```python
from build123d import *

# Parameters (mm, degrees)
CROQUIS1_W              = 82
CROQUIS1_H              = 90.5
CROQUIS1_R              = 1.4
SALIENTE_EXTRUIR1_DEPTH = 1.5
CROQUIS1_3_W            = 82
CROQUIS1_3_H            = 2
SALIENTE_EXTRUIR2_DEPTH = 9.31
SALIENTE_EXTRUIR3_START = 9.31
CROQUIS1_4_W            = 82
CROQUIS1_4_H            = 7.5
CROQUIS1_4_R            = 1.4
CROQUIS1_4_H_2          = 2
SALIENTE_EXTRUIR3_DEPTH = 2
CROQUIS2_R              = 1.5
CROQUIS2_R_2            = 1.6
CORTAR_EXTRUIR1_DEPTH   = 1.5
CROQUIS3_W              = 48
CROQUIS3_H              = 7.5
CORTAR_EXTRUIR2_DEPTH   = 87.58467604
REDONDEO1_R             = 5
REDONDEO2_R             = 3


with BuildPart() as part:
    # Croquis1 → Saliente-Extruir1 (new body)
    with BuildSketch(Plane(origin=(0, 0, 0), x_dir=(1, 0, 0), z_dir=(0, 1, 0))):
        with Locations((2.5, 28.755)):
            Rectangle(CROQUIS1_W, CROQUIS1_H)
        with Locations(Location((-25.63, 31.995, 0), (0, 0, 270))):
            Circle(CROQUIS1_R, mode=Mode.SUBTRACT)
        with Locations(Location((25.63, 31.995, 0), (0, 0, 270))):
            Circle(CROQUIS1_R, mode=Mode.SUBTRACT)
    extrude(amount=SALIENTE_EXTRUIR1_DEPTH)

    # Croquis2 → Cortar-Extruir1 (cut)
    with BuildSketch(Plane(origin=(0, 1.5, 0), x_dir=(1, 0, 0), z_dir=(0, 1, 0))):
        with Locations(Location((-23.4, -1.495, 0), (0, 0, 270))):
            Circle(CROQUIS2_R)
        with Locations(Location((23.4, -1.495, 0), (0, 0, 270))):
            Circle(CROQUIS2_R)
        with Locations(Location((0, 30.505, 0), (0, 0, 270))):
            Circle(CROQUIS2_R)
        with Locations(Location((-20.86, 57.715, 0), (0, 0, 270))):
            Circle(CROQUIS2_R_2)
        with Locations(Location((20.86, 57.715, 0), (0, 0, 270))):
            Circle(CROQUIS2_R_2)
        with Locations(Location((20.86, 15.995, 0), (0, 0, 270))):
            Circle(CROQUIS2_R_2)
        with Locations(Location((-20.86, 15.995, 0), (0, 0, 270))):
            Circle(CROQUIS2_R_2)
    extrude(amount=-CORTAR_EXTRUIR1_DEPTH, mode=Mode.SUBTRACT)


with BuildPart() as body_2:
    # Croquis1<3> → Saliente-Extruir2 (new body)
    with BuildSketch(Plane(origin=(0, 0, 0), x_dir=(1, 0, 0), z_dir=(0, 1, 0))):
        with Locations((2.5, -17.495)):
            Rectangle(CROQUIS1_3_W, CROQUIS1_3_H)
    extrude(amount=SALIENTE_EXTRUIR2_DEPTH)

    # Croquis1<4> → Saliente-Extruir3 (add)
    # profile 1 of 2: a face of its own
    with BuildSketch(Plane(origin=(0, 0, 0), x_dir=(1, 0, 0), z_dir=(0, 1, 0)).offset(SALIENTE_EXTRUIR3_START)):
        with Locations((2.5, -22.245)):
            Rectangle(CROQUIS1_4_W, CROQUIS1_4_H)
        with Locations(Location((-19, -21.995, 0), (0, 0, 270))):
            Circle(CROQUIS1_4_R, mode=Mode.SUBTRACT)
        with Locations(Location((39, -21.995, 0), (0, 0, 270))):
            Circle(CROQUIS1_4_R, mode=Mode.SUBTRACT)
    # profile 2 of 2: a face of its own
    with BuildSketch(Plane(origin=(0, 0, 0), x_dir=(1, 0, 0), z_dir=(0, 1, 0)).offset(SALIENTE_EXTRUIR3_START)):
        with Locations((2.5, -17.495)):
            Rectangle(CROQUIS1_4_W, CROQUIS1_4_H_2)
    extrude(amount=SALIENTE_EXTRUIR3_DEPTH)

    # Combinar1: union part
    add(part.part)

    # Croquis3 → Cortar-Extruir2 (cut, through all)
    with BuildSketch(Plane(origin=(0, 11.31, 0), x_dir=(1, 0, 0), z_dir=(0, 1, 0))):
        Polygon((-18.5, -25.995), (-28, -16.495), (-38.5, -16.495), (-38.5, -25.995), align=None)
        Polygon((-28, -16.495), (-38.5, -5.995), (-38.5, -16.495), align=None)
        with Locations((10.5, -22.245)):
            Rectangle(CROQUIS3_W, CROQUIS3_H)
        Polygon((-38.5, 54.005), (-18.5, 74.005), (-38.5, 74.005), align=None)
        Polygon((23.5, 74.005), (43.5, 54.005), (43.5, 74.005), align=None)
    extrude(amount=-CORTAR_EXTRUIR2_DEPTH, mode=Mode.SUBTRACT)

    # Redondeo1
    redondeo1_edges = [body_2.edges().sort_by_distance(p)[0] for p in [
        (23.5, 0.75, -74.005),
        (43.5, 0.75, -54.005),
        (-38.5, 0.75, 5.995),
        (-18.5, 0.75, -74.005),
        (-38.5, 0.75, -54.005),
    ]]
    fillet(redondeo1_edges, radius=REDONDEO1_R)

    # Redondeo2
    redondeo2_edges = [body_2.edges().sort_by_distance(p)[0] for p in [
        (-18.5, 10.31, 25.995),
        (43.5, 10.31, 25.995),
        (34.5, 10.31, 18.495),
        (-13.5, 10.31, 25.995),
        (-13.5, 10.31, 18.495),
        (34.5, 10.31, 25.995),
    ]]
    fillet(redondeo2_edges, radius=REDONDEO2_R)


solid = body_2.part
```
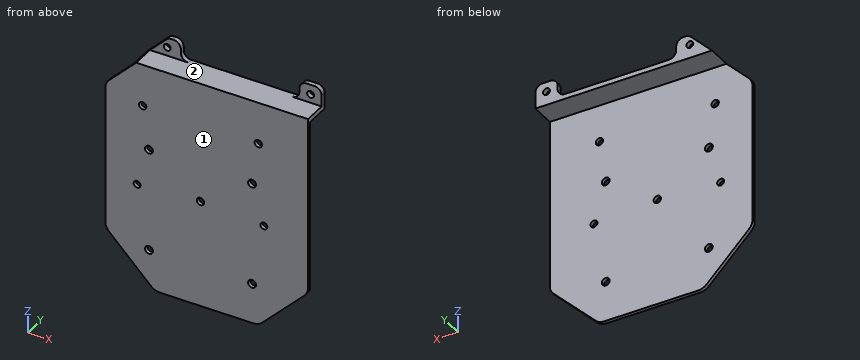
Input: part model. Units: mm. Frame: model coordinates. Face numbers are marked on the shaded views. Give positions to 0.01 mm unless a question says otherwise; leave off trailing zeros. Order: outer loops, then holes, each group sorted by start corner. A loop starts at its lowest first (then second) coordinate and runs counter-clockwise, first axis right, second up.
1. Cut plane A-A (x = 39). Return loops of the section in (y, z) (3 decimals).
Computed:
outline: (0, -58.505) - (1.5, -58.505) - (1.5, 16.495) - (11.31, 16.495) - (11.31, 20.595) - (9.31, 20.595) - (9.31, 18.495) - (0, 18.495) - close; (9.31, 23.395) - (11.31, 23.395) - (11.31, 25.995) - (9.31, 25.995) - close
2. Pin query (flat end, axial travel): pin 1 Ø3 at (x, z) = (-20.86, -15.995) entering from -Y; pin 2 Ø4.5 at (x, z) = (39, 21.995) entering from -Y; pin 3 Ø3 at (x, y) = (3, 9.5) entering from +Z (3 decimals); pin 4 Ø0.8 at (y, z) = (10.5, 22.5) entering from -X (3 decimals). Return the tip coordinate at first contact, or that it passes through.
Computed:
pin 1: passes through
pin 2: stops at y = 9.31
pin 3: stops at z = 18.495
pin 4: stops at x = -22.395
3. Cut plane D-D (y = 6.75). Return loops of the section in (x, z) (3 decimals), and give its area (3 significant figures).
Computed:
outline: (-28, 16.495) - (43.5, 16.495) - (43.5, 18.495) - (-26, 18.495) - close
area: 141 mm2
4. Cut plane C-C (z = -38). Return loops of the section in (x, y).
Computed:
outline: (-38.5, 0) - (43.5, 0) - (43.5, 1.5) - (-38.5, 1.5) - close
5. Draft query along X for the marked faces 1 and 2. Return one class per face: released by +X, released by -X, zero draft, split by the parting line, or undercut.
Computed:
face 1: zero draft
face 2: undercut
6. Line query: probe 1 along Z at (x, y) = (-25, 8) (3 decimals); probe 2 along Y at (x, z) = (-20.5, -55.5); probe 3 along X at (y, z) = (10.5, 17.5) (3 decimals). Output: solid intervals per line, ascending.
Computed:
probe 1: z = 16.495 to 18.495
probe 2: y = 0 to 1.5
probe 3: x = -26.995 to 43.5
7. Cut plane B-B (x = -3). Return loops of the section in (y, z) (3 decimals), and give its area (3 significant figures).
Computed:
outline: (0, -74.005) - (1.5, -74.005) - (1.5, 16.495) - (11.31, 16.495) - (11.31, 18.495) - (0, 18.495) - close
area: 158 mm2
